from build123d import *

# Parameters (mm, degrees)
F0_R         = 1.5
F0_W         = 3
F0_H         = 13.7437733207
F0_H_2       = 1.2562266793
F1_DEPTH     = 4
F2_DEPTH     = 19
F3_R         = 7.49999
F4_R         = 2.5
F5_DEPTH     = 28.851
F6_T1_DEPTH  = 4
F6_T6_DEPTH  = 3
F6_T11_DEPTH = 9.4292074699
F6_T18_DEPTH = 9.4292074699
F6_T25_DEPTH = 3
F6_T30_DEPTH = 9.4292074699
F6_T37_DEPTH = 9.4292074699
F6_T44_DEPTH = 3
F7_T1_DEPTH  = 17.2196709514
F7_T3_DEPTH  = 29


# Not quite as in the source:
# - a fillet or chamfer that OpenCascade refuses, or shapes differently, is made with other operations: its cross-section is extruded or revolved along the edge and cut away or added
# - a fillet or chamfer is up to 0.001 mm smaller than in the source, because OpenCascade refuses the exact size


with BuildPart() as f1:
    # F0 (on Top) → F1 (new body)
    with BuildSketch(Plane.XY):
        Polygon((-12.9930239742, 7.1134486855), (-21.35, 7.1134486855), (-21.35, -7.1134486855), (21.35, -7.1134486855), (21.35, 7.1134486855), (12.9930239742, 7.1134486855), (7.5, 7.1134486855), (7.5, -6.6303246352), (4.5, -6.6303246352), (4.5, 7.1134486855), (1.5, 7.1134486855), (1.5, -6.6303246352), (-1.5, -6.6303246352), (-1.5, 7.1134486855), (-4.5, 7.1134486855), (-4.5, -6.6303246352), (-7.5, -6.6303246352), (-7.5, 7.1134486855), align=None)
        with Locations((-16.25, 0)):
            Circle(F0_R, mode=Mode.SUBTRACT)
        with Locations((16.25, 0)):
            Circle(F0_R, mode=Mode.SUBTRACT)
        Polygon((-12.9930239742, 10.3696753648), (-12.9930239742, 7.1134486855), (-7.5, 7.1134486855), (-7.5, 8.3696753648), (-4.5, 8.3696753648), (-1.5, 8.3696753648), (1.5, 8.3696753648), (4.5, 8.3696753648), (7.5, 8.3696753648), (7.5, 7.1134486855), (12.9930239742, 7.1134486855), (12.9930239742, 10.3696753648), align=None)
        with Locations((-6, 0.2415620252)):
            Rectangle(F0_W, F0_H)
        with Locations((-6, 7.7415620252)):
            Rectangle(F0_W, F0_H_2)
        with Locations((-3, 7.7415620252)):
            Rectangle(F0_W, F0_H_2)
        Polygon((-1.5, 8.3696753648), (-1.5, 7.1134486855), (0, 7.1134486855), (1.5, 7.1134486855), (1.5, 8.3696753648), align=None)
        Polygon((0, 7.1134486855), (-1.5, 7.1134486855), (-1.5, -6.6303246352), (1.5, -6.6303246352), (1.5, 7.1134486855), align=None)
        with Locations((3, 7.7415620252)):
            Rectangle(F0_W, F0_H_2)
        with Locations((6, 0.2415620252)):
            Rectangle(F0_W, F0_H)
        with Locations((6, 7.7415620252)):
            Rectangle(F0_W, F0_H_2)
    extrude(amount=F1_DEPTH)

    # F0 (on Top) → F2 (join)
    with BuildSketch(Plane.XY):
        with Locations((-6, 0.2415620252)):
            Rectangle(F0_W, F0_H)
        with Locations((-6, 7.7415620252)):
            Rectangle(F0_W, F0_H_2)
        Polygon((-1.5, 8.3696753648), (-1.5, 7.1134486855), (0, 7.1134486855), (1.5, 7.1134486855), (1.5, 8.3696753648), align=None)
        Polygon((0, 7.1134486855), (-1.5, 7.1134486855), (-1.5, -6.6303246352), (1.5, -6.6303246352), (1.5, 7.1134486855), align=None)
        with Locations((6, 0.2415620252)):
            Rectangle(F0_W, F0_H)
        with Locations((6, 7.7415620252)):
            Rectangle(F0_W, F0_H_2)
    extrude(amount=F2_DEPTH)

    # F3 (radius 7.5 in the source; OpenCascade refuses exactly that, so slightly less here)
    f3_edges = [f1.edges().sort_by_distance(p)[0] for p in [
        (-6, -6.630325, 19),
        (0, -6.630325, 19),
        (6, -6.630325, 19),
        (6, 8.369675, 19),
        (0, 8.369675, 19),
        (-6, 8.369675, 19),
    ]]
    fillet(f3_edges, radius=F3_R)

    # F4 (on face) → F5 (cut, through all)
    with BuildSketch(Plane(origin=(-7.5, 0, 0), x_dir=(0, -1, 0), z_dir=(-1, 0, 0))):
        with Locations((-0.8696753648, 11.5)):
            Circle(F4_R)
    extrude(amount=-F5_DEPTH, mode=Mode.SUBTRACT)

    # F6: chamfer of 2.5 on 5 edges, made by hand

    # F6_s2 → F6_t1 (join)
    with BuildSketch(Plane.XY):
        Polygon((12.9930239742, 9.6134486855), (15.4930239742, 7.1134486855), (12.9930239742, 7.1134486855), align=None)
        Polygon((-15.4930239742, 7.1134486855), (-12.9930239742, 9.6134486855), (-12.9930239742, 7.1134486855), align=None)
    extrude(amount=F6_T1_DEPTH)


with BuildPart() as f6_tool4:
    # F6_s5 → F6_t6 (new body)
    with BuildSketch(Plane.YZ.offset(-7.5)):
        Polygon((8.3696753648, 6.5), (10.8696753648, 4), (8.3696753648, 4), align=None)
    extrude(amount=F6_T6_DEPTH)

    split(bisect_by=Plane.XZ.offset(-10.3696753648), keep=Keep.TOP)


with BuildPart() as f1_1:
    add(f1.part)

    # F6_t3: union F6_tool4
    add(f6_tool4.part)


with BuildPart() as f6_tool9:
    # F6_s10 → F6_t11 (new body)
    with BuildSketch(Plane.YZ.offset(-7.5)):
        Polygon((8.3696753648, 6.5), (10.8696753648, 4), (8.3696753648, 4), align=None)
    extrude(amount=F6_T11_DEPTH)

    split(bisect_by=Plane.XZ.offset(-10.3696753648), keep=Keep.TOP)

    split(bisect_by=Plane.YZ.offset(-1.5), keep=Keep.TOP)

    split(bisect_by=Plane.YZ.offset(1.5), keep=Keep.BOTTOM)


with BuildPart() as f1_2:
    add(f1_1.part)

    # F6_t8: union F6_tool9
    add(f6_tool9.part)


with BuildPart() as f6_tool16:
    # F6_s17 → F6_t18 (new body)
    with BuildSketch(Plane.YZ.offset(-7.9292074699)):
        Polygon((10.8696753648, 4), (8.3696753648, 6.5), (8.3696753648, 4), align=None)
    extrude(amount=F6_T18_DEPTH)

    split(bisect_by=Plane.YZ.offset(-7.5), keep=Keep.TOP)

    split(bisect_by=Plane.YZ.offset(-4.5), keep=Keep.BOTTOM)

    split(bisect_by=Plane.XZ.offset(-10.3696753648), keep=Keep.TOP)


with BuildPart() as f1_3:
    add(f1_2.part)

    # F6_t15: union F6_tool16
    add(f6_tool16.part)


with BuildPart() as f6_tool23:
    # F6_s24 → F6_t25 (new body)
    with BuildSketch(Plane.YZ.offset(-1.5)):
        Polygon((10.8696753648, 4), (8.3696753648, 6.5), (8.3696753648, 4), align=None)
    extrude(amount=F6_T25_DEPTH)

    split(bisect_by=Plane.XZ.offset(-10.3696753648), keep=Keep.TOP)


with BuildPart() as f1_4:
    add(f1_3.part)

    # F6_t22: union F6_tool23
    add(f6_tool23.part)


with BuildPart() as f6_tool28:
    # F6_s29 → F6_t30 (new body)
    with BuildSketch(Plane.YZ.offset(-1.5)):
        Polygon((10.8696753648, 4), (8.3696753648, 6.5), (8.3696753648, 4), align=None)
    extrude(amount=F6_T30_DEPTH)

    split(bisect_by=Plane.XZ.offset(-10.3696753648), keep=Keep.TOP)

    split(bisect_by=Plane.YZ.offset(4.5), keep=Keep.TOP)

    split(bisect_by=Plane.YZ.offset(7.5), keep=Keep.BOTTOM)


with BuildPart() as f1_5:
    add(f1_4.part)

    # F6_t27: union F6_tool28
    add(f6_tool28.part)


with BuildPart() as f6_tool35:
    # F6_s36 → F6_t37 (new body)
    with BuildSketch(Plane.YZ.offset(-1.9292074699)):
        Polygon((10.8696753648, 4), (8.3696753648, 6.5), (8.3696753648, 4), align=None)
    extrude(amount=F6_T37_DEPTH)

    split(bisect_by=Plane.XZ.offset(-10.3696753648), keep=Keep.TOP)

    split(bisect_by=Plane.YZ.offset(-1.5), keep=Keep.TOP)

    split(bisect_by=Plane.YZ.offset(1.5), keep=Keep.BOTTOM)


with BuildPart() as f1_6:
    add(f1_5.part)

    # F6_t34: union F6_tool35
    add(f6_tool35.part)


with BuildPart() as f6_tool42:
    # F6_s43 → F6_t44 (new body)
    with BuildSketch(Plane.YZ.offset(4.5)):
        Polygon((10.8696753648, 4), (8.3696753648, 6.5), (8.3696753648, 4), align=None)
    extrude(amount=F6_T44_DEPTH)

    split(bisect_by=Plane.XZ.offset(-10.3696753648), keep=Keep.TOP)


with BuildPart() as f1_7:
    add(f1_6.part)

    # F6_t41: union F6_tool42
    add(f6_tool42.part)

    # F7: fillet of radius 5 on 6 edges, made by hand

    # F7_s2 → F7_t1 (cut)
    with BuildSketch(Plane.XY.offset(-6.6098354757)):
        with BuildLine():
            ThreePointArc((10.3490897839, 10.3696753648), (11.7240685831, 10.1769025595), (12.9930239742, 9.6134486855))
            Line((12.9930239742, 9.6134486855), (12.9930239742, 10.3696753648))
            Line((12.9930239742, 10.3696753648), (10.3490897839, 10.3696753648))
        make_face()
        with BuildLine():
            ThreePointArc((-10.3490897839, 10.3696753648), (-11.7240685831, 10.1769025595), (-12.9930239742, 9.6134486855))
            Line((-12.9930239742, 9.6134486855), (-12.9930239742, 10.3696753648))
            Line((-12.9930239742, 10.3696753648), (-10.3490897839, 10.3696753648))
        make_face()
    extrude(amount=F7_T1_DEPTH, mode=Mode.SUBTRACT)

    # F7_s4 → F7_t3 (cut)
    with BuildSketch(Plane.XY.offset(-12.5)):
        with BuildLine():
            ThreePointArc((-21.35, 2.1134486855), (-19.8855339059, 5.6489825915), (-16.35, 7.1134486855))
            Line((-16.35, 7.1134486855), (-21.35, 7.1134486855))
            Line((-21.35, 7.1134486855), (-21.35, 2.1134486855))
        make_face()
        with BuildLine():
            ThreePointArc((-16.35, -7.1134486855), (-19.8855339059, -5.6489825915), (-21.35, -2.1134486855))
            Line((-21.35, -2.1134486855), (-21.35, -7.1134486855))
            Line((-21.35, -7.1134486855), (-16.35, -7.1134486855))
        make_face()
        with BuildLine():
            ThreePointArc((21.35, -2.1134486855), (19.8855339059, -5.6489825915), (16.35, -7.1134486855))
            Line((16.35, -7.1134486855), (21.35, -7.1134486855))
            Line((21.35, -7.1134486855), (21.35, -2.1134486855))
        make_face()
        with BuildLine():
            ThreePointArc((16.35, 7.1134486855), (19.8855339059, 5.6489825915), (21.35, 2.1134486855))
            Line((21.35, 2.1134486855), (21.35, 7.1134486855))
            Line((21.35, 7.1134486855), (16.35, 7.1134486855))
        make_face()
    extrude(amount=F7_T3_DEPTH, mode=Mode.SUBTRACT)


solid = f1_7.part
Can you work these out from the model? Positions are in its coordinate system, mm. A direction names the side the tool comes from. Give positions to 0.01 mm unless a question says otherwise; leave off trailing zeros. Write each loop counter-clockwise with the first axis right and the second up, starting at its lowest first coordinate (ties: lowest second). Pieces come first, ordered by that corner, then holes. Notation, with made-up numbers: M 73.25,-38.5 L 81.25,-38.5 A22 cw 81.25,-1.5 Z; hole C 47.25,-29.75 d8. An arc over 180 degrees is marked long. Answer in a Markdown table with one row per item. Add a question column.
Item 1: Please list where these lines run through material, in increasing order: L1, parallel to X at y = 8.25, z = 8; L2, parallel to Y at x = 16.25, z = 2.8; L3, parallel to Z at x = -19, y = -3.
Item 2: Imagine slicing it at B-B, the plane x = 17. Write out the boundary of the cut face in (y, z).
Item 3: Imagine slicing it at A-A, the plane z = 7.5. Write out the boundary of the cut face in (x, y).
Item 4: For pin 1 Ø0.9 at (x, z) = (5.5, 10) entering from +Y; pin 2 Ø0.9 at (x, z) = (-5.5, 8) entering from -Y; pin 3 Ø4.5 at (y, z) = (0.87, 11.5) entering from +X; pin 4 Ø3 at (y, z) = (2.5, 12.5) entering from +X, each with a flat end and sliding along its axis, tell me the tip position at first contact or that it passes through.
Item 5: Imagine slicing it at C-C, the plane y = 2.75. Write out the boundary of the cut face in (x, z), plus the area to 3 significant figures.
Item 6: On a 3-axis mill with a long thin cutter (end or side, diameter ignored), from which of +Z, -Z, +X, -X, +Y, -Y can I reach the whole of each face in a straight line? I mean faces 1 (the flat face through (0, -6.63, 8)), 2 (the flat face through (-7.5, 2, 8)), 3 (the flat face through (16, 7.113, 2)). Say none if no direction works.
Item 7: We'd pull the mould along X, two halves only. Please class faces 4 (the flat face through (4.5, 2, 8)), 5 (the cylindrical face through (-5.979, -4.492, 16.745)), 6 (the cylindrical face through (19.924, -5.61, 1.972)): released by +X, released by -X, zero draft, split by the parting line, or undercut.
Evaluation:
| question | item | result |
|---|---|---|
| 1 | L1 | x = -7.5 to -4.5, -1.5 to 1.5, 4.5 to 7.5 |
| 1 | L2 | y = -7.11 to -1.5, 1.5 to 7.11 |
| 1 | L3 | z = 0 to 4 |
| 2 | outline | M -7.07,0 L -1.3,0 L -1.3,4 L -7.07,4 Z; M 1.3,0 L 7.07,0 L 7.07,4 L 1.3,4 Z |
| 3 | outline | M -7.5,-6.63 L -4.5,-6.63 L -4.5,8.37 L -7.5,8.37 Z; M -1.5,-6.63 L 1.5,-6.63 L 1.5,8.37 L -1.5,8.37 Z; M 4.5,-6.63 L 7.5,-6.63 L 7.5,8.37 L 4.5,8.37 Z |
| 4 | pin 1 | stops at y = 8.37 |
| 4 | pin 2 | stops at y = -6.63 |
| 4 | pin 3 | passes through |
| 4 | pin 4 | stops at x = 7.5 |
| 5 | outline | M -21.31,0 L 21.31,0 L 21.31,4 L 7.5,4 L 7.5,9.85 L 4.5,9.85 L 4.5,4 L 1.5,4 L 1.5,9.85 L -1.5,9.85 L -1.5,4 L -4.5,4 L -4.5,9.85 L -7.5,9.85 L -7.5,4 L -21.31,4 Z; M -7.5,13.15 L -4.5,13.15 L -4.5,18.76 L -7.5,18.76 Z; M -1.5,13.15 L 1.5,13.15 L 1.5,18.76 L -1.5,18.76 Z; M 4.5,13.15 L 7.5,13.15 L 7.5,18.76 L 4.5,18.76 Z |
| 5 | area | 274 mm² |
| 6 | face 1 | +Z, +X, -X, -Y |
| 6 | face 2 | +Z, -X, +Y, -Y |
| 6 | face 3 | +Z, -Z, +X, +Y |
| 7 | face 4 | undercut |
| 7 | face 5 | zero draft |
| 7 | face 6 | released by +X |
